```python
from build123d import *

# Parameters (mm, degrees)
BOSS_EXTRUDE1_DEPTH = 5.08
SKETCH3_R           = 3.175
CUT_EXTRUDE1_DEPTH  = 5.08


with BuildPart() as part:
    # Sketch1 → Boss-Extrude1 (new body)
    with BuildSketch(Plane(origin=(0, 0, 0), x_dir=(1, 0, 0), z_dir=(0, 1, 0))):
        with BuildLine():
            Line((381, 0), (381, 381))
            ThreePointArc((381, 381), (269.407683632, 111.592316368), (0, 0))
            Line((0, 0), (381, 0))
        make_face()
    extrude(amount=BOSS_EXTRUDE1_DEPTH)

    # Sketch3 → Cut-Extrude1 (cut)
    with BuildSketch(Plane(origin=(0, 5.08, 0), x_dir=(1, 0, 0), z_dir=(0, 1, 0))):
        with Locations(Location((101.6, 6.35, 0), (0, 0, 270))):
            Circle(SKETCH3_R)
        with Locations(Location((374.65, 279.4, 0), (0, 0, 270))):
            Circle(SKETCH3_R)
        with Locations(Location((368.3, 12.7, 0), (0, 0, 270))):
            Circle(SKETCH3_R)
        with Locations(Location((279.4, 101.6, 0), (0, 0, 270))):
            Circle(SKETCH3_R)
        with Locations(Location((203.2, 48.26, 0), (0, 0, 270))):
            Circle(SKETCH3_R)
        with Locations(Location((332.74, 177.8, 0), (0, 0, 270))):
            Circle(SKETCH3_R)
        with Locations(Location((228.6, 12.7, 0), (0, 0, 270))):
            Circle(SKETCH3_R)
        with Locations(Location((368.3, 152.4, 0), (0, 0, 270))):
            Circle(SKETCH3_R)
    extrude(amount=-CUT_EXTRUDE1_DEPTH, mode=Mode.SUBTRACT)


solid = part.part
```
The model under review builds one solid part; all positions refer to its coordinate system, in mm. Give positions to 0.01 mm unless a question says otherwise; leave off trailing zeros. Write each loop counter-clockwise with the first axis right and the second up, starting at its lowest first coordinate (ties: lowest second). Pieces come first, ordered by that corner, then holes. Notation, with made-up numbers: (18, -19) -> (77, -19) arc R25 ccw to (77, 20) -> close; hole circle Ø11 at (28.5, 11). An arc over 180 degrees is marked (long way). Answer in a Markdown table with one row per item.
1) For L1, parallel to Z at x = 203.2, y = 3.85 (3 decimals); L2, parallel to X at y = 4, z = -177.8 (3 decimals); L3, parallel to X at y = 0.3, z = -152, list the stretches that pass through material, from the lowest coordinate up. Write a range as [from, to].
Worked answers:
| item | result |
|---|---|
| L1 | [-58.71, -51.435], [-45.085, 0] |
| L2 | [322.29, 329.565], [335.915, 381] |
| L3 | [304.5, 365.15], [371.45, 381] |
2) Clearance check with a flat-ended pin moving along its axis: P1, Ø5.5, axis at x = 279.4, z = -101.6, coming from the -Y side (1 decimal). State where the tip first meets the part, or that it passes through.
Worked answers:
| item | result |
|---|---|
| P1 | through |
3) Add section C-C on x = 132.5. State the section outline as (y, z) points, plus the area to 3 significant figures.
Worked answers:
| item | result |
|---|---|
| outline | (0, -23.78) -> (5.08, -23.78) -> (5.08, 0) -> (0, 0) -> close |
| area | 121 mm² |
4) Add section A-A on y = 3.75. Count the separate pieces of the cut face and the enclosed holes in it, plus the area to 3 significant figures.
Worked answers:
| item | result |
|---|---|
| separate pieces | 1 |
| enclosed holes | 8 |
| area | 30,900 mm² |
